Input: part model. Units: mm. Frame: model coordinates. Coordinates: 2 decimals unless noted, no trailing zeros. Loops run counter-clockwise (first coordinate to the right, second up) from the corner with the lowest first, then second, coordinate; pieces in that order, holes last. Notation, with made-up numbers: (-39, 52.25) -> (11, 52.25) arc R29 cw to (11, 88.25) -> close; hole circle Ø11 at (26, 29.25). An arc over 180 degrees is marked (long way). Answer as a JSON object with one key per item and string values.
from build123d import *

# Parameters (mm, degrees)
F0_W     = 150
F0_H     = 150
F0_W_2   = 140
F0_H_2   = 140
F1_DEPTH = 1.4
F2_R     = 2.1
F3_R     = 0.7
F4_R     = 2.1
F5_R     = 2.1
F6_R     = 0.7
F7_R     = 2.1
F8_R     = 0.7
F9_R     = 0.7


with BuildPart() as f1:
    # F0 (on Top) → F1 (new body)
    with BuildSketch(Plane.XY):
        Rectangle(F0_W, F0_H)
        Rectangle(F0_W_2, F0_H_2, mode=Mode.SUBTRACT)
    extrude(amount=F1_DEPTH)

    # F2
    f2_edges = [f1.edges().sort_by_distance(p)[0] for p in [
        (75, 75, 0.7),
    ]]
    fillet(f2_edges, radius=F2_R)

    # F3
    f3_edges = [f1.edges().sort_by_distance(p)[0] for p in [
        (70, 70, 0.7),
    ]]
    fillet(f3_edges, radius=F3_R)

    # F4
    f4_edges = [f1.edges().sort_by_distance(p)[0] for p in [
        (-75, 75, 0.7),
    ]]
    fillet(f4_edges, radius=F4_R)

    # F5
    f5_edges = [f1.edges().sort_by_distance(p)[0] for p in [
        (-75, -75, 0.7),
    ]]
    fillet(f5_edges, radius=F5_R)

    # F6
    f6_edges = [f1.edges().sort_by_distance(p)[0] for p in [
        (-70, -70, 0.7),
    ]]
    fillet(f6_edges, radius=F6_R)

    # F7
    f7_edges = [f1.edges().sort_by_distance(p)[0] for p in [
        (75, -75, 0.7),
    ]]
    fillet(f7_edges, radius=F7_R)

    # F8
    f8_edges = [f1.edges().sort_by_distance(p)[0] for p in [
        (70, -70, 0.7),
    ]]
    fillet(f8_edges, radius=F8_R)

    # F9
    f9_edges = [f1.edges().sort_by_distance(p)[0] for p in [
        (-70, 70, 0.7),
    ]]
    fillet(f9_edges, radius=F9_R)


solid = f1.part
1. Section query A-A (z = 0.8). Return loops of the section in (x, y), plus the area to 3 significant figures.
Reply:
{"outline": "(-75, -72.9) arc R2.1 ccw to (-72.9, -75) -> (72.9, -75) arc R2.1 ccw to (75, -72.9) -> (75, 72.9) arc R2.1 ccw to (72.9, 75) -> (-72.9, 75) arc R2.1 ccw to (-75, 72.9) -> close; hole (-70, -69.3) arc R0.7 ccw to (-69.3, -70) -> (69.3, -70) arc R0.7 ccw to (70, -69.3) -> (70, 69.3) arc R0.7 ccw to (69.3, 70) -> (-69.3, 70) arc R0.7 ccw to (-70, 69.3) -> close", "area": "2,900 mm2"}
2. Line query: line 1 along Y through (x, z) = (63, 0.25). Output: solid intervals per line, ascending.
Reply:
{"line 1": "y = -75 to -70, 70 to 75"}
3. Section query B-B (y = 55). Return loops of the section in (x, z), plus the area to 3 significant figures.
Reply:
{"outline": "(-75, 0) -> (-70, 0) -> (-70, 1.4) -> (-75, 1.4) -> close; (70, 0) -> (75, 0) -> (75, 1.4) -> (70, 1.4) -> close", "area": "14.0 mm2"}
